Drawing for the job (mm, zero at the part's lowest x, y, z). A direction names the side the tool comes from. Give positions to 0.01 mm unless a question says otherwise; leave off trailing zeros. Write each loop counter-clockwise with the first axis right and the second up, starting at its lowest first coordinate (ties: lowest second). Pieces come first, ordered by that corner, then holes.
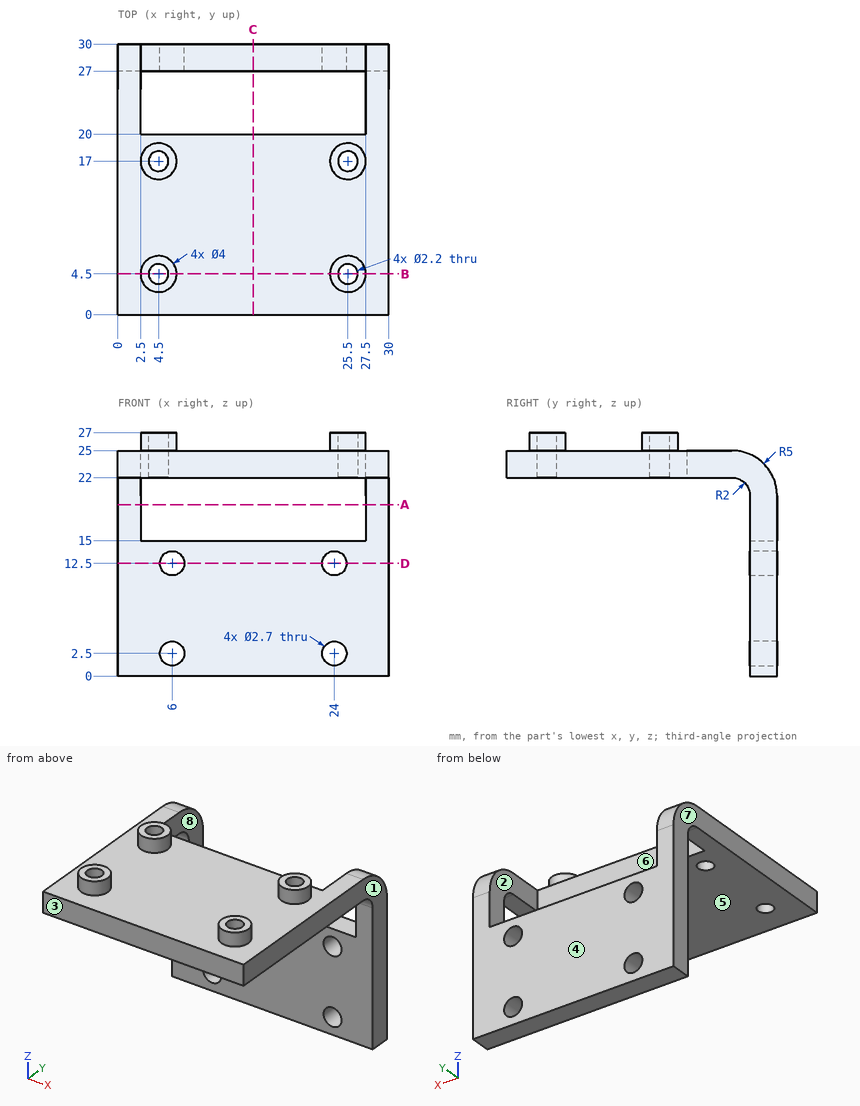
1. Slice it at C-C, the plane x = 15. Write the cut outline in (y, z).
Calculated:
outline: (0, 22) - (20, 22) - (20, 25) - (0, 25) - close; (27, 0) - (30, 0) - (30, 15) - (27, 15) - close
2. Pin check, flat tips, straight feed: P1, Ø3.5, axis at x = 20.5, z = 24, coming from the +Y side; P2, Ø8, axis at x = 22, z = 15.5, coming from the -Y side; P3, Ø3.5, axis at x = 4.5, y = 17, coming from the +Z side; P4, Ø3.5, axis at x = 12.5, y = 28.5, coming from the +Z side. Stop position of each tip, or through.
Calculated:
P1: stops at y = 20
P2: stops at y = 27
P3: stops at z = 27
P4: stops at z = 15
3. Slice it at B-B, the plane y = 4.5. Write the cut outline in (x, z), and give its area (3 significant figures).
Calculated:
outline: (0, 22) - (3.4, 22) - (3.4, 27) - (2.5, 27) - (2.5, 25) - (0, 25) - close; (5.6, 22) - (24.4, 22) - (24.4, 27) - (23.5, 27) - (23.5, 25) - (6.5, 25) - (6.5, 27) - (5.6, 27) - close; (26.6, 22) - (30, 22) - (30, 25) - (27.5, 25) - (27.5, 27) - (26.6, 27) - close
area: 84.0 mm2
4. Pull direction X, two halves, no side cores. Call the marked faces 1, 2 and 3: +X half, -X half, draft (parallel to the pull), parting line (faces both ways), or undercut.
Calculated:
face 1: +X half
face 2: undercut
face 3: draft
5. Slice it at D-D, the plane z = 12.5. Write the cut outline in (x, y).
Calculated:
outline: (0, 27) - (4.65, 27) - (4.65, 30) - (0, 30) - close; (7.35, 27) - (22.65, 27) - (22.65, 30) - (7.35, 30) - close; (25.35, 27) - (30, 27) - (30, 30) - (25.35, 30) - close
6. Probe probe 1 along Y at (x, z) = (25.5, 24.75); probe 2 along X at (y, z) = (28.2, 12.5); probe 3 along X at (y, z) = (27.75, 16). List the from-to ranges inside material, lowest first.
Calculated:
probe 1: y = 0 to 3.4, 5.6 to 15.9, 18.1 to 20
probe 2: x = 0 to 4.65, 7.35 to 22.65, 25.35 to 30
probe 3: x = 0 to 2.5, 27.5 to 30
7. Slice it at A-A, the plane z = 19. Write the cut outline in (x, y).
Calculated:
outline: (0, 27) - (2.5, 27) - (2.5, 30) - (0, 30) - close; (27.5, 27) - (30, 27) - (30, 30) - (27.5, 30) - close
8. Which spindle directions (+Z, -Z, +X, -X, +Y, -Y) get a long thin tool onto all of the face, cutting with end or side? Do the marked faces 4, 5, 6, 7 and 8. Say none if no direction does.
Calculated:
face 4: +Z, -Z, +X, -X, +Y
face 5: -Z, +X, -X, -Y
face 6: +Z, -Z, +Y
face 7: +Z, -Z, -X, +Y, -Y
face 8: +Z, +Y
